Design review of the part shown in the three views and the two pictorial views. Dimensions are in mm from the part's minimum x, y and z. Round coordinates to 2 decimals unless told otherwise and drop trailing zeros. Loops run counter-clockwise (first coordinate to the right, second up) from the corner with the lowest first, then second, coordinate; pieces in that order, holes last.
1) Insertion check: pin 1 (1.5 mm diameter, centred on x = 16.5, z = 2.5, fed in from +Y); pin 2 (0.9 mm diameter, centred on x = 18.5, z = 3, fed in from -Y); pin 3 (0.9 mm diameter, centred on y = 19.5, z = 3, fed in from +X). Each pin has a flat end and moves straight along its axis. Give the tip position at first contact, or say it passes through.
2) Take a section at D-D (z = 0.5). State the section outline as (x, y) points.
3) Mouldability with a two-part tool opening along X and no side actions: class the marked faces 1 and 2 as pulls with the +X half, pulls with the -X half, needs draft (parallel to the pull), parting line crosses it, or undercut.
4) Take a section at A-A (y = 28.5). State the section outline as (x, z) points.
5) Take a section at C-C (y = 4). State the section outline as (x, z) points, then the cut area to 3 significant figures.
6) Take a section at B-B (x = 33). State the section outline as (y, z) points, then the cut area to 3 significant figures.
7) Wall thickness on L1, parallel to Y at x = 19.5, z = 1.1; L2, parallel to X at y = 24.5, z = 1.8; L3, parallel to Y at x = 24.5, z = 2.35: over which ranges is each line inside the solid? List them lowest first.
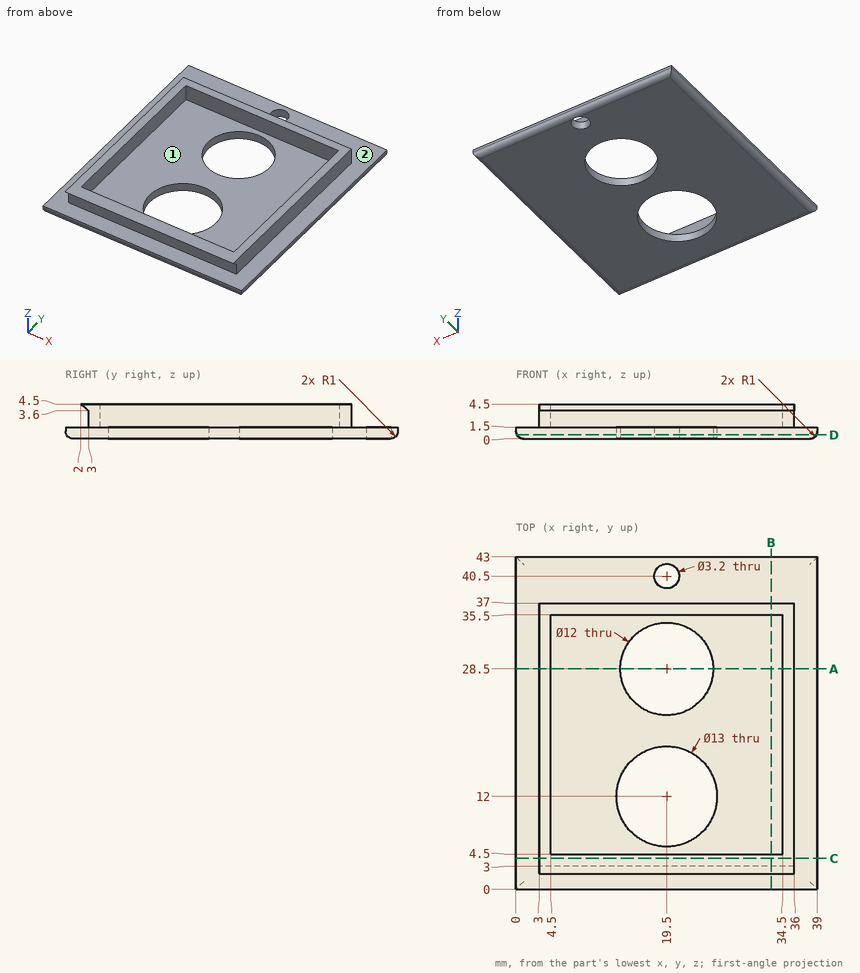
Response:
1. pin 1: stops at y = 37
1. pin 2: stops at y = 3
1. pin 3: stops at x = 36
2. outline: (0.13, 0.13) - (38.87, 0.13) - (38.87, 42.87) - (0.13, 42.87) - close; hole circle Ø13 at (19.5, 12); hole circle Ø12 at (19.5, 28.5); hole circle Ø3.2 at (19.5, 40.5)
3. face 1: undercut
3. face 2: needs draft
4. outline: (0, 1) arc R1 ccw to (1, 0) - (13.5, 0) - (13.5, 1.5) - (4.5, 1.5) - (4.5, 4.5) - (3, 4.5) - (3, 1.5) - (0, 1.5) - close; (25.5, 0) - (38, 0) arc R1 ccw to (39, 1) - (39, 1.5) - (36, 1.5) - (36, 4.5) - (34.5, 4.5) - (34.5, 1.5) - (25.5, 1.5) - close
5. outline: (0, 1) arc R1 ccw to (1, 0) - (38, 0) arc R1 ccw to (39, 1) - (39, 1.5) - (36, 1.5) - (36, 4.5) - (3, 4.5) - (3, 1.5) - (0, 1.5) - close
5. area: 157 mm2
6. outline: (0, 1) arc R1 ccw to (1, 0) - (42, 0) arc R1 ccw to (43, 1) - (43, 1.5) - (37, 1.5) - (37, 4.5) - (35.5, 4.5) - (35.5, 1.5) - (4.5, 1.5) - (4.5, 4.5) - (2, 4.5) - (3, 3.6) - (3, 1.5) - (0, 1.5) - close
6. area: 73.5 mm2
7. L1: y = 0 to 5.5, 18.5 to 22.5, 34.5 to 38.9, 42.1 to 43
7. L2: x = 3 to 4.5, 34.5 to 36
7. L3: y = 3 to 4.5, 35.5 to 37
